from build123d import *

# Parameters (mm, degrees)
F3_DEPTH = 25
F4_SIZE  = 1
F5_R     = 2.1
F6_DEPTH = 6


with BuildPart() as f1:
    # F0 (on Top) → F1 (revolve)
    with BuildSketch(Plane.XY):
        with BuildLine():
            Line((0, 15), (0, 0))
            Line((0, 0), (36, 0))
            Line((36, 0), (36, 4))
            Line((36, 4), (20, 4))
            ThreePointArc((20, 4), (19.7071067812, 3.2928932188), (19, 3))
            ThreePointArc((19, 3), (18.2928932188, 3.2928932188), (18, 4))
            Line((18, 4), (18, 6))
            Line((18, 6), (6, 6))
            Line((6, 6), (6, 15))
            Line((6, 15), (0, 15))
        make_face()
    revolve(axis=Axis((18, 0, 0), (-1, 0, 0)))

    # F2 (on face) → F3 (cut)
    with BuildSketch(Plane(origin=(0, 0, 0), x_dir=(0, -1, 0), z_dir=(-1, 0, 0))):
        with BuildLine():
            Line((23.4234053642, 26.5963438079), (-25.4426617175, 26.5963438079))
            Line((-25.4426617175, 26.5963438079), (-25.4426617175, 13))
            Line((-25.4426617175, 13), (-7.4833147735, 13))
            ThreePointArc((-7.4833147735, 13), (0, 15), (7.4833147735, 13))
            Line((7.4833147735, 13), (23.4234053642, 13))
            Line((23.4234053642, 13), (23.4234053642, 26.5963438079))
        make_face()
        with BuildLine():
            ThreePointArc((7.4833147735, 13), (0, 15), (-7.4833147735, 13))
            Line((-7.4833147735, 13), (7.4833147735, 13))
        make_face()
    extrude(amount=-F3_DEPTH, mode=Mode.SUBTRACT)

    # F4
    f4_edges = [f1.edges().sort_by_distance(p)[0] for p in [
        (0, 0, -15),
        (0, 0, 13),
        (36, -4, 0),
    ]]
    chamfer(f4_edges, length=F4_SIZE)

    # F5 (on face) → F6 (cut)
    with BuildSketch(Plane(origin=(0, 0, 0), x_dir=(0, -1, 0), z_dir=(-1, 0, 0))):
        with Locations((0, -9)):
            Circle(F5_R)
    extrude(amount=-F6_DEPTH, mode=Mode.SUBTRACT)


solid = f1.part
CAD build for the part. Positions are in the model's coordinates, mm. A direction names the side the tool comes from. Give positions to 0.01 mm unless a question says otherwise; leave off trailing zeros. Write each loop counter-clockwise with the first axis right and the second up, starting at its lowest first coordinate (ties: lowest second). Pieces come first, ordered by that corner, then holes. Notation, with made-up numbers: (81, 87) -> (92, 87) arc R22 cw to (92, 100) -> close; hole circle Ø4 at (65, -2.75). An arc over 180 degrees is marked (long way). Return JSON: item names as keys, results as strings.
Item 1: Tool access for faces 1 (the flat face through (36, 0, 0)), 2 (the cylindrical face through (27.395, -0.867, 3.905)): list every direction of +Z, -Z, +X, -X, +Y, -Y with a clear straight run to the whole face (end or side of a thin tool).
Answer below:
{"face 1": "+Z, -Z, +X, +Y, -Y", "face 2": "+X"}
Item 2: Band-saw the part on A-A (x = 18.5). List the corners of the cut face in (y, z), then the cut area to 3 significant figures.
Answer below:
{"outline": "circle Ø6.27 at (0, 0)", "area": "30.9 mm2"}
Item 3: Drop flat-ended pins along their axis: pin 1 (2 mm diameter, centred on x = 18.5, z = 3.5, fed in from -Y); pin 2 (10 mm diameter, centred on x = 30.5, z = 3.5, fed in from -Y); pin 3 (8 mm diameter, centred on x = 17, y = -8, fed in from -Z). Give the stop position or say it passes through.
Answer below:
{"pin 1": "stops at y = -5.39", "pin 2": "stops at y = -4", "pin 3": "stops at z = -4.47"}
Item 4: Two-plate mould, pull along Y, no slides. Class faces 3 (the flat face through (0, 0, -1)), 4 (the cylindrical face through (2.958, 0.273, -6.918)), 5 (the cylindrical face through (3.46, 0.55, -14.99)): +Y half, -Y half, draft (parallel to the pull), parting line (faces both ways), or undercut.
Answer below:
{"face 3": "draft", "face 4": "undercut", "face 5": "parting line"}
Item 5: Drill centre lines: probe 1 along Z at (x, y) = (3.9, 0); probe 2 along Y at (x, z) = (30.5, 0); probe 3 along X at (y, z) = (-3, -5). Where is each one in solid material? Low to high.
Answer below:
{"probe 1": "z = -15 to -11.1, -6.9 to 13", "probe 2": "y = -4 to 4", "probe 3": "x = 0 to 18"}
